from build123d import *

# Parameters (mm, degrees)
SKETCH_1_W          = 60
SKETCH_1_H          = 60
EXTRUDE_1_DEPTH     = 2
M4X0_7_1_D          = 3.3
M4X0_7_1_DEPTH      = 11.5
M4X0_7_1_TIP        = 0.991420021
CUT_EXTRUDE_1_DEPTH = 80


with BuildPart() as part:
    # ｽｹｯﾁ1 → ﾎﾞｽ - 押し出し1 (new body)
    with BuildSketch(Plane.XY):
        Rectangle(SKETCH_1_W, SKETCH_1_H)
    extrude(amount=EXTRUDE_1_DEPTH)

    # M4x0.7 ねじ穴1
    with Locations(Plane(origin=(22, 22, 0), x_dir=(-1, 0, 0), z_dir=(0, 0, -1))):
        with Locations((0, 0), (0, -44), (44, -44), (44, 0)):
            Hole(M4X0_7_1_D / 2, depth=M4X0_7_1_DEPTH)
            with Locations((0, 0, -(M4X0_7_1_DEPTH + M4X0_7_1_TIP / 2))):  # 118° drill point
                Cone(0, M4X0_7_1_D / 2, M4X0_7_1_TIP, mode=Mode.SUBTRACT)

    # ｽｹｯﾁ4 → ｶｯﾄ - 押し出し1 (cut)
    with BuildSketch(Plane(origin=(0, 0, 0), x_dir=(-1, 0, 0), z_dir=(0, 0, -1))):
        Polygon((-30, -30), (-30, -20), (-20, -30), align=None)
        Polygon((-24.998553068, 25.001446932), (-30, 20), (-30, 30), (-20, 30), align=None)
        Polygon((30, 30), (20, 30), (30, 20), align=None)
        Polygon((30, -30), (30, -20), (20, -30), align=None)
    extrude(amount=-CUT_EXTRUDE_1_DEPTH, mode=Mode.SUBTRACT)


solid = part.part
Could you check a few things on this model? Use its own coordinates, in mm. Give positions to 0.01 mm unless a question says otherwise; leave off trailing zeros. Order: outer loops, then holes, each group sorted by start corner. A loop starts at its lowest first (then second) coordinate and runs counter-clockwise, first axis right, second up.
Item 1: If we section it at A-A, the plane x = 22: Write out the boundary of the cut face in (y, z), plus the area to 3 significant figures.
Item 2: I'm going to push flat-ended pins straight in: pin 1 (2 mm diameter, centred on x = -22, y = 22, fed in from +Z); pin 2 (12 mm diameter, centred on x = 14.5, y = -11.5, fed in from -Z); pin 3 (1 mm diameter, centred on y = 23, z = 1.5, fed in from -X). Where does each tip first touch, or does it pass through?
Item 3: I need wall thicknesses on line 1 (Y direction, x = -22, z = 0.6); line 2 (X direction, y = 23.5, z = 0.1); line 3 (X direction, y = 23, z = 1). Which ranges of each line are inside material? Lowest first, please.
Item 4: If we section it at C-C, the plane z = 1.35: Write out the boundary of the cut face in (x, y).
Item 5: If we mould it in two halves opening along Y, with no side actions, what happens to faces 1 (the face through (25, -25, 1)), 2 (the face through (20.784, -20.885, 1.014)), 3 (the face through (0, 0, 0))? For each: pulls with the +Y half, pulls with the -Y half, needs draft (parallel to the pull), parting line crosses it, or undercut.
Values:
1. outline: (-28, 0) - (-23.65, 0) - (-23.65, 2) - (-28, 2) - close; (-20.35, 0) - (20.35, 0) - (20.35, 2) - (-20.35, 2) - close; (23.65, 0) - (28, 0) - (28, 2) - (23.65, 2) - close
1. area: 98.8 mm2
2. pin 1: passes through
2. pin 2: stops at z = 0
2. pin 3: stops at x = -27.5
3. line 1: y = -28 to -23.65, -20.35 to 20.35, 23.65 to 28
3. line 2: x = -26.5 to -22.69, -21.31 to 21.31, 22.69 to 26.5
3. line 3: x = -27 to -23.31, -20.69 to 20.69, 23.31 to 27
4. outline: (-30, -20) - (-20, -30) - (20, -30) - (30, -20) - (30, 20) - (20, 30) - (-20, 30) - (-30, 20) - close; hole circle Ø3.3 at (-22, -22); hole circle Ø3.3 at (-22, 22); hole circle Ø3.3 at (22, -22); hole circle Ø3.3 at (22, 22)
5. face 1: pulls with the -Y half
5. face 2: undercut
5. face 3: needs draft
